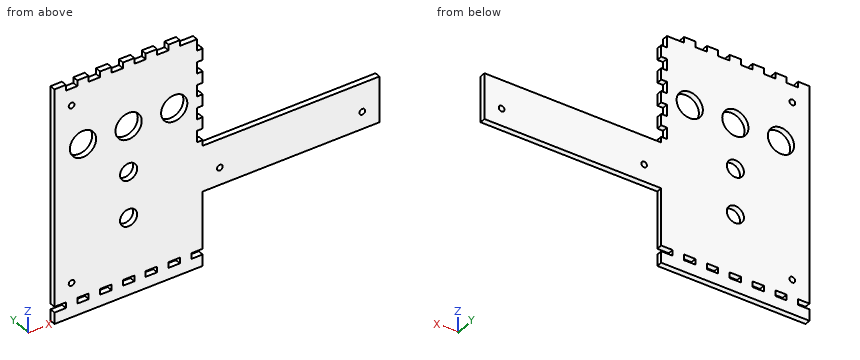
from build123d import *

# Parameters (mm, degrees)
PAD_DEPTH       = 2.5
SKETCH001_W     = 10
SKETCH001_H     = 5
POCKET_DEPTH    = 5.001
SKETCH002_R     = 2.5
POCKET001_DEPTH = 5.001
SKETCH003_W     = 10
SKETCH003_H     = 5
SKETCH003_W_2   = 20
POCKET002_DEPTH = 5.001
SKETCH004_W     = 5
SKETCH004_H     = 10
POCKET003_DEPTH = 5.001
SKETCH005_R     = 11.5
POCKET004_DEPTH = 5.001
SKETCH006_R     = 7.5
POCKET005_DEPTH = 5.001


with BuildPart() as part:
    # Sketch → Pad (new body, symmetric)
    with BuildSketch(Plane.XZ):
        Polygon((-65, 102.5), (65, 102.5), (65, 2.5), (220, 2.5), (220, -37.5), (65, -37.5), (65, -102.5), (-65, -102.5), align=None)
    extrude(amount=PAD_DEPTH, both=True)

    # Sketch001 (on Face10 of Pad) → Pocket (cut, through all)
    with BuildSketch(Plane.XZ.offset(2.5)):
        with Locations((-60, -90)):
            Rectangle(SKETCH001_W, SKETCH001_H)
        with Locations((-40, -90)):
            Rectangle(SKETCH001_W, SKETCH001_H)
        with Locations((-20, -90)):
            Rectangle(SKETCH001_W, SKETCH001_H)
        with Locations((0, -90)):
            Rectangle(SKETCH001_W, SKETCH001_H)
        with Locations((20, -90)):
            Rectangle(SKETCH001_W, SKETCH001_H)
        with Locations((40, -90)):
            Rectangle(SKETCH001_W, SKETCH001_H)
        with Locations((60, -90)):
            Rectangle(SKETCH001_W, SKETCH001_H)
    extrude(amount=-POCKET_DEPTH, mode=Mode.SUBTRACT)

    # Sketch002 (on Face5 of Pocket) → Pocket001 (cut, through all)
    with BuildSketch(Plane.XZ.offset(2.5)):
        with Locations((-50, 82.5)):
            Circle(SKETCH002_R)
        with Locations((-50, -72.5)):
            Circle(SKETCH002_R)
        with Locations((80, -22.5)):
            Circle(SKETCH002_R)
        with Locations((205, -22.5)):
            Circle(SKETCH002_R)
    extrude(amount=-POCKET001_DEPTH, mode=Mode.SUBTRACT)

    # Sketch003 (on Face5 of Pocket001) → Pocket002 (cut, through all)
    with BuildSketch(Plane.XZ.offset(2.5)):
        with Locations((-50, 100)):
            Rectangle(SKETCH003_W, SKETCH003_H)
        with Locations((-30, 100)):
            Rectangle(SKETCH003_W, SKETCH003_H)
        with Locations((-10, 100)):
            Rectangle(SKETCH003_W, SKETCH003_H)
        with Locations((10, 100)):
            Rectangle(SKETCH003_W, SKETCH003_H)
        with Locations((30, 100)):
            Rectangle(SKETCH003_W, SKETCH003_H)
        with Locations((55, 100)):
            Rectangle(SKETCH003_W_2, SKETCH003_H)
    extrude(amount=-POCKET002_DEPTH, mode=Mode.SUBTRACT)

    # Sketch004 (on Face4 of Pocket002) → Pocket003 (cut, through all)
    with BuildSketch(Plane.XZ.offset(2.5)):
        with Locations((62.5, 92.5)):
            Rectangle(SKETCH004_W, SKETCH004_H)
        with Locations((62.5, 72.5)):
            Rectangle(SKETCH004_W, SKETCH004_H)
        with Locations((62.5, 52.5)):
            Rectangle(SKETCH004_W, SKETCH004_H)
        with Locations((62.5, 32.5)):
            Rectangle(SKETCH004_W, SKETCH004_H)
        with Locations((62.5, 12.5)):
            Rectangle(SKETCH004_W, SKETCH004_H)
    extrude(amount=-POCKET003_DEPTH, mode=Mode.SUBTRACT)

    # Sketch005 (on Face4 of Pocket003) → Pocket004 (cut, through all)
    with BuildSketch(Plane.XZ.offset(2.5)):
        with Locations((-40, 45)):
            Circle(SKETCH005_R)
        with Locations((0, 45)):
            Circle(SKETCH005_R)
        with Locations((40, 45)):
            Circle(SKETCH005_R)
    extrude(amount=-POCKET004_DEPTH, mode=Mode.SUBTRACT)

    # Sketch006 (on Face4 of Pocket004) → Pocket005 (cut, through all)
    with BuildSketch(Plane.XZ.offset(2.5)):
        with Locations((0, 5)):
            Circle(SKETCH006_R)
        with Locations((0, -35)):
            Circle(SKETCH006_R)
    extrude(amount=-POCKET005_DEPTH, mode=Mode.SUBTRACT)


solid = part.part
Build history of the part. All positions in model axes, mm. Coordinates: 2 decimals unless noted, no trailing zeros. Order: outer loops, then holes, each group sorted by start corner. A loop starts at its lowest first (then second) coordinate and runs counter-clockwise, first axis right, second up. Notation, with made-up numbers: M 52.25,-32 L 87.25,-32 A23 ccw 87.25,-7 Z; hole C 28,0 d9. An arc over 180 degrees is marked long. One line per question, with ' | ' between items. Start each with the question number.
Q1. Saw through at C-C (y = 1.6). Count the separate pieces of the cut face and the enclosed holes in it, then the cut area to 3 significant figures.
Q2. Saw through at A-A (x = -40). List the corners of the cut face in (y, z).
Q3. Saw through at D-D (z = -83). List the corners of the cut face in (x, y).
Q4. Probe L1, parallel to Z at x = 40, y = 1.1; L2, parallel to Z at x = 0, y = 1.25; L3, parallel to Z at x = 80, y = -1.1. List the from-to ranges inside material, lowest first. Write a range as from..to.
Q5. Saw through at B-B (x = 0). List the corners of the cut face in (y, z).
Q6. Flat gauge pins, fed straight in: pin 1 Ø1.5 at (y, z) = (0.5, -96.5) entering from +X; pin 2 Ø5 at (x, z) = (89, 6.5) entering from -Y; pin 3 Ø2.5 at (y, z) = (-1, -91) entering from +X; pin 4 Ø1 at (y, z) = (1, 32.5) entering from +X. Where does each tip first touch, or does it go through?
Check values:
1) separate pieces: 1 | enclosed holes: 14 | area: 30,200 mm2
2) outline: M -2.5,-102.5 L 2.5,-102.5 L 2.5,-92.5 L -2.5,-92.5 Z; M -2.5,-87.5 L 2.5,-87.5 L 2.5,33.5 L -2.5,33.5 Z; M -2.5,56.5 L 2.5,56.5 L 2.5,102.5 L -2.5,102.5 Z
3) outline: M -65,-2.5 L 65,-2.5 L 65,2.5 L -65,2.5 Z
4) L1: z = -102.5..-92.5, -87.5..33.5, 56.5..102.5 | L2: z = -102.5..-92.5, -87.5..-42.5, -27.5..-2.5, 12.5..33.5, 56.5..102.5 | L3: z = -37.5..-25, -20..2.5
5) outline: M -2.5,-102.5 L 2.5,-102.5 L 2.5,-92.5 L -2.5,-92.5 Z; M -2.5,-87.5 L 2.5,-87.5 L 2.5,-42.5 L -2.5,-42.5 Z; M -2.5,-27.5 L 2.5,-27.5 L 2.5,-2.5 L -2.5,-2.5 Z; M -2.5,12.5 L 2.5,12.5 L 2.5,33.5 L -2.5,33.5 Z; M -2.5,56.5 L 2.5,56.5 L 2.5,102.5 L -2.5,102.5 Z
6) pin 1: stops at x = 65 | pin 2: passes through | pin 3: stops at x = 55 | pin 4: stops at x = 60
